Autodesk Inventor part; units mm, degrees
ref_plane "YZ Plane" through (0, 0, 0) normal (1, 0, 0) x (0, 1, 0)
ref_plane "XZ Plane" through (0, 0, 0) normal (0, 1, 0) x (-1, 0, 0)
ref_plane "XY Plane" through (0, 0, 0) normal (0, 0, 1) x (1, 0, 0)
sketch "Sketch1" plane through (0, 0, 0) normal (0, 1, 0) x (-1, 0, 0)
  line L0 (-40.259, 19.431) -> (40.259, 19.431)
  line L1 (40.259, 19.431) -> (40.259, -19.431)
  line L2 (40.259, -19.431) -> (-40.259, -19.431)
  line L3 (-40.259, -19.431) -> (-40.259, 19.431)
  line L4 (-40.259, 11.811) -> (-38.735, 11.811)
  line L5 (-38.735, 11.811) -> (-38.735, 10.287)
  line L6 (-38.735, 10.287) -> (-40.259, 10.287)
  line L7 (-40.259, 10.287) -> (-40.259, 11.811)
  line L8 (40.259, 11.811) -> (38.735, 11.811)
  line L9 (38.735, 11.811) -> (38.735, 10.287)
  line L10 (38.735, 10.287) -> (40.259, 10.287)
  line L11 (40.259, 10.287) -> (40.259, 11.811)
  point P0 (0, 0)
  point P1 (40.259, 0)
  point P2 (0, -19.431)
  point P3 (0, 0)
  dimension "d0" = 80.518
  dimension "d1" = 38.862
  dimension "d20" = 1.524
  dimension "d21" = 7.62
extrude "Extrusion1" add sketch "Sketch1" against normal blind 80.518 contours L0 L1 L8 L9 L10 L2 L3 L6 L5 L4
sketch "Sketch2" plane through (0, 0, 0) normal (0, 1, 0) x (-1, 0, 0)
  line L0 (-30.48, -11.811) -> (30.48, -11.811)
  line L1 (30.48, -11.811) -> (30.48, 11.811)
  line L2 (30.48, 11.811) -> (-30.48, 11.811)
  line L3 (-30.48, 11.811) -> (-30.48, -11.811)
  line L4 (40.259, -19.431) -> (-40.259, -19.431)
  line L5 (-40.259, 19.431) -> (40.259, 19.431)
  point P0 (0, 0)
  point P1 (0, 11.811)
  point P2 (-30.48, 0)
  dimension "d4" = 60.96
  dimension "d5" = 23.622
extrude "Extrusion2" cut sketch "Sketch2" against normal blind 14.478
sketch "Sketch3" plane through (0, -80.518, 0) normal (0, -1, 0) x (1, 0, 0)
  line L0 (-31.75, -12.7) -> (31.75, -12.7)
  line L1 (31.75, -12.7) -> (31.75, 12.7)
  line L2 (31.75, 12.7) -> (-31.75, 12.7)
  line L3 (-31.75, 12.7) -> (-31.75, -12.7)
  point P0 (0, 0)
  point P1 (0, -12.7)
  point P2 (-31.75, 0)
  dimension "d10" = 63.5
  dimension "d11" = 25.4
extrude "Extrusion3" cut sketch "Sketch3" against normal blind 14.478
sketch "Sketch4" plane through (40.259, 0, 19.431) normal (0, 0, 1) x (-1, 0, 0)
  line L0 (65.3415, 20.828) -> (15.1765, 20.828)
  line L1 (15.1765, 20.828) -> (15.1765, 61.214)
  line L2 (15.1765, 61.214) -> (65.3415, 61.214)
  line L3 (65.3415, 61.214) -> (65.3415, 20.828)
  line L4 (0, 0) -> (80.518, 0)
  point P0 (40.259, 0)
  point P1 (40.259, 0)
  point P2 (40.259, 20.828)
  dimension "d15" = 20.828
  dimension "d16" = 40.386
  dimension "d17" = 50.165
extrude "Extrusion4" cut sketch "Sketch4" against normal blind 27.178
fillet "Fillet1" radius 5.08 12 edges at (30.48, -7.239, 11.811) (30.48, -7.239, -11.811) (-30.48, -7.239, -11.811) (-30.48, -7.239, 11.811) (-31.75, -73.279, -12.7) (-31.75, -73.279, 12.7) (31.75, -73.279, 12.7) (31.75, -73.279, -12.7) (-25.0825, -20.828, 5.842) (25.0825, -20.828, 5.842) (25.0825, -61.214, 5.842) (-25.0825, -61.214, 5.842)
fillet "Fillet1" radius 7.62 4 edges at (-40.259, -40.259, 19.431) (-40.259, -40.259, -19.431) (40.259, -40.259, 19.431) (40.259, -40.259, -19.431)
fillet "Fillet2" radius 0.254 16 edges at (38.0273, -80.518, -17.1993) (0, -80.518, -19.431) (-38.0273, -80.518, -17.1993) (-40.259, -80.518, -0.7623) (40.259, -80.518, -0.7623) (0, -80.518, 19.431) (-38.0273, -80.518, 17.1993) (38.0273, -80.518, 17.1993) (0, 0, 19.431) (-38.0273, 0, 17.1993) (38.0273, 0, 17.1993) (38.0273, 0, -17.1993) (0, 0, -19.431) (-38.0273, 0, -17.1993) (-40.259, 0, -0.7623) (40.259, 0, -0.7623)
properties part number "T9 Passenger Section"
The model under review builds one solid part; all positions refer to its coordinate system, in mm. A direction names the side the tool comes from. Round coordinates to 2 decimals unless told otherwise and drop trailing zeros. Order: outer loops, then holes, each group sorted by start corner. A loop starts at its lowest first (then second) coordinate and runs counter-clockwise, first axis right, second up. Notation, with made-up numbers: (7.5, 67.5) -> (50.5, 67.5) arc R22 cw to (50.5, 102.5) -> close; hole circle Ø10 at (-9.75, -12.5). An arc over 180 degrees is marked (long way). Return JSON: item names as keys, results as strings.
1. Insertion check: P1, Ø8, axis at x = 5.5, z = 1.5, coming from the +Y side; P2, Ø0.8, axis at x = 40, y = -32.5, coming from the -Z side; P3, Ø1.2, axis at y = -48.5, z = 10.5, coming from the -X side; P4, Ø0.8, axis at x = 39.5, y = -60, coming from the +Z side. Each pin has a flat end and moves straight along its axis. Give the tip position at first contact, or say it passes through.
Answer block:
{"P1": "stops at y = -14.48", "P2": "stops at z = -14.91", "P3": "stops at x = -40.26", "P4": "stops at z = 15.85"}
2. For L1, parallel to Y at x = 8.5, z = -2; L2, parallel to Y at x = -7.5, z = 13.5; L3, parallel to X at y = -26, z = 10, list the stretches that pass through material, from the lowest coordinate up. Write a range as [from, to].
Answer block:
{"L1": "y = [-66.04, -61.21], [-20.83, -14.48]", "L2": "y = [-80.52, -61.21], [-20.83, 0]", "L3": "x = [-40.26, -25.08], [25.08, 40.26]"}
3. Take a section at D-D (x = -9.5). Write out the cut boundary in (y, z), then the cut area to 3 significant figures.
Answer block:
{"outline": "(-80.52, -19.18) arc R0.25 ccw to (-80.26, -19.43) -> (-0.25, -19.43) arc R0.25 ccw to (0, -19.18) -> (0, -11.81) -> (-14.48, -11.81) -> (-14.48, 11.81) -> (0, 11.81) -> (0, 19.18) arc R0.25 ccw to (-0.25, 19.43) -> (-20.83, 19.43) -> (-20.83, -7.75) -> (-61.21, -7.75) -> (-61.21, 19.43) -> (-80.26, 19.43) arc R0.25 ccw to (-80.52, 19.18) -> (-80.52, 12.7) -> (-66.04, 12.7) -> (-66.04, -12.7) -> (-80.52, -12.7) -> close", "area": "1,320 mm²"}
4. For faces 1 (the face through (30.302, -73.178, -11.173)), 2 (the face through (0, -61.214, 6)), 3 (the face through (0, -14.478, 0)), 4 (the face through (-40.259, -40, -1)), list the 3-axis set-ups (+Z, -Z, +X, -X, +Y, -Y) from which the entire face can be reached by the end or side of a thin tool; tool diameter is ignored.
Answer block:
{"face 1": "-Y", "face 2": "+Z", "face 3": "+Y", "face 4": "+Z, -Z, -X, +Y, -Y"}
5. The part is to be moulded in two halves that separate along Y. For faces 5 (the face through (23.56, -22.28, 5.65)), 6 (the face through (-38.086, -40.819, -17.14)), 7 (the face through (1, 0, 13)), 8 (the face through (0, -66.04, 0)), say which applies: +Y half, -Y half, draft (parallel to the pull), parting line (faces both ways), or undercut.
Answer block:
{"face 5": "undercut", "face 6": "draft", "face 7": "+Y half", "face 8": "-Y half"}
